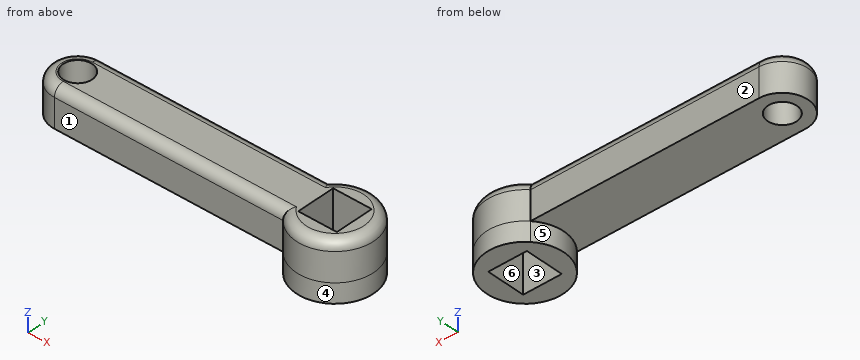
Autodesk Inventor part; units mm, degrees
ref_plane "YZ Plane" through (0, 0, 0) normal (1, 0, 0) x (0, 1, 0)
ref_plane "XZ Plane" through (0, 0, 0) normal (0, 1, 0) x (-1, 0, 0)
ref_plane "XY Plane" through (0, 0, 0) normal (0, 0, 1) x (1, 0, 0)
sketch "Sketch1" plane through (0, 0, 0) normal (0, 0, 1) x (1, 0, 0)
  circle A0 centre (-39.9943, 0) radius 2.25
  arc A1 (-5.0436, -3.25) -> (-5.0436, 3.25) centre (0, 0) ccw
  line L0 (3, 3) -> (3, -3)
  line L1 (3, -3) -> (-3, -3)
  line L2 (-3, -3) -> (-3, 3)
  line L3 (-3, 3) -> (3, 3)
  line L4 (-3, 3) -> (3, 3)
  line L5 (-3, -3) -> (3, -3)
  line L6 (-39.9943, -4) -> (-4.4721, -4)
  line L7 (-4.4721, 4) -> (-39.9943, 4)
  arc A2 (-39.9943, 4) -> (-39.9943, -4) centre (-39.9943, 0) ccw
  point P0 (0, 3)
  point P1 (-19.9972, 0)
extrude "Extrusion1" add sketch "Sketch1" along normal blind 6
sketch "Sketch5" plane through (0, 0, 0) normal (0, 0, -1) x (-1, 0, 0)
  circle A0 centre (0, 0) radius 6
  arc A1 (4.4721, 4) -> (4.4721, -4) centre (0, 0) ccw
  line L0 (-3, -3) -> (-3, 3)
  line L1 (-3, 3) -> (3, 3)
  line L2 (3, 3) -> (3, -3)
  line L3 (3, -3) -> (-3, -3)
  point P0 (2.804, -2.804)
  point P1 (5.0436, -3.25)
  point P2 (5.0436, 3.25)
  point P3 (0, -3)
extrude "Extrusion5" add sketch "Sketch5" along normal blind 3
fillet "Fillet2" radius 1.5 4 edges at (-22.2332, -4, 6) (-43.9943, 0, 6) (-22.2332, 4, 6) (6, 0, 6)
scale "Scale1" factors (0.5, 0.5, 0.5) then translate (-11.1166, 2, 0) bodies 1
properties part number "crankshaft"
Input: part model. Units: mm. Frame: model coordinates. Face numbers are marked on the shaded views. A direction names the side the tool comes from. Give positions to 0.01 mm unless a question says otherwise; leave off trailing zeros. Order: outer loops, then holes, each group sorted by start corner. A loop starts at its lowest first (then second) coordinate and runs counter-clockwise, first axis right, second up. Notation, with made-up numbers: (34.25, -32) - (80.25, -32) arc R17 ccw to (80.25, -28) - close; hole circle Ø2 at (-34, -21). An arc over 180 degrees is marked (long way). Answer as a JSON object with one key per item and string values. Group by question number.
Q1. Line query: probe 1 along X at (y, z) = (2.5, 1.5); probe 2 along Y at (x, z) = (-17.5, 1.1); probe 3 along Z at (x, y) = (-29.5, 0.75). Output: solid intervals per line, ascending.
Q2. Set-up query: the marked faces 1, 2 and 3. Return all of +Z, -Z, +X, -X, +Y, -Y with unobstructed straight access to the full face (end or side cutting, diameter ignored); none if empty.
Q3. Cut plane C-C, the plane x = -20.5. Output: boundary loops of the cut face in (y, z), then the cut area to 3 significant figures.
Q4. Cut plane D-D, the plane z = 1.9. Output: boundary loops of the cut face in (x, y) (3 decimals), then the cut area to 3 significant figures.
Q5. Mould query, pull axis X, two halves, no side actions, for the marked faces 4, 5 and 6. Classes: pulls with the +X half, pulls with the -X half, needs draft (parallel to the pull), parting line crosses it, or undercut.
Q6. Cut plane B-B, the plane z = -1.2. Output: boundary loops of the cut face in (x, y), then the cut area to 3 significant figures.
Q7. First-contact query: pin 1 Ø1.5 at (y, z) = (0, -0.5) entering from +X; pin 2 Ø2.5 at (x, z) = (-26, 1.5) entering from -Y; pin 3 Ø2 at (x, y) = (-20.5, 1.5) entering from -Z. Flat tips, straight axial feed; report the tip coordinate or a pass-through.
Q8. Cut plane A-A, the plane y = 2. Output: boundary loops of the cut face in (x, z), then the cut area to 3 significant figures.
Results:
{
 "1": {"probe 1": "-33.05 to -32.12, -30.11 to -12.62, -9.62 to -8.16", "probe 2": "0 to 4", "probe 3": "0 to 3"},
 "2": {"face 1": "+Z, -Z, -X, -Y", "face 2": "+Z, -Z, -X, +Y", "face 3": "+Z, -Z"},
 "3": {"outline": "(0, 0) - (4, 0) - (4, 2.25) arc R0.75 ccw to (3.25, 3) - (0.75, 3) arc R0.75 ccw to (0, 2.25) - close", "area": "11.8 mm^2"},
 "4": {"outline": "(-31.114, 0) - (-13.353, 0) arc R3 ccw (long way) to (-13.353, 4) - (-31.114, 4) arc R2 ccw to start; hole circle Ø2.25 at (-31.114, 2); hole (-12.617, 0.5) - (-9.617, 0.5) - (-9.617, 3.5) - (-12.617, 3.5) - close", "area": "90.5 mm^2"},
 "5": {"face 4": "parting line crosses it", "face 5": "pulls with the -X half", "face 6": "undercut"},
 "6": {"outline": "circle Ø6 at (-11.12, 2); hole (-12.62, 0.5) - (-9.62, 0.5) - (-9.62, 3.5) - (-12.62, 3.5) - close", "area": "19.3 mm^2"},
 "7": {"pin 1": "x = -8.39", "pin 2": "y = 0", "pin 3": "z = 0"},
 "8": {"outline": "(-33.11, 0) - (-32.24, 0) - (-32.24, 3) - (-32.36, 3) arc R0.75 ccw to (-33.11, 2.25) - close; (-29.99, 0) - (-14.12, 0) - (-14.12, -1.5) - (-12.62, -1.5) - (-12.62, 3) - (-29.99, 3) - close; (-9.62, -1.5) - (-8.12, -1.5) - (-8.12, 2.25) arc R0.75 ccw to (-8.87, 3) - (-9.62, 3) - close", "area": "63.5 mm^2"}
}
